from build123d import *

# Parameters (mm, degrees)
F0_R     = 12.7
F1_DEPTH = 12.7
F2_R     = 3.2385
F3_DEPTH = 12.7
F4_R     = 1.905
F5_DEPTH = 12.7


with BuildPart() as f1:
    # F0 (on Front) → F1 (new body)
    with BuildSketch(Plane.XZ):
        Circle(F0_R)
    extrude(amount=F1_DEPTH)

    # F2 (on face) → F3 (cut)
    with BuildSketch(Plane.XZ.offset(12.7)):
        Circle(F2_R)
    extrude(amount=-F3_DEPTH, mode=Mode.SUBTRACT)

    # F4 (on face) → F5 (join)
    with BuildSketch(Plane.XZ.offset(12.7)):
        with Locations((-8.480146, 3.001869)):
            Circle(F4_R)
        with Locations((-5.475456, -7.13747)):
            Circle(F4_R)
        with Locations((5.096128, -7.413068)):
            Circle(F4_R)
        with Locations((8.625037, 2.555942)):
            Circle(F4_R)
        with Locations((0.234438, 8.992727)):
            Circle(F4_R)
    extrude(amount=F5_DEPTH)


solid = f1.part
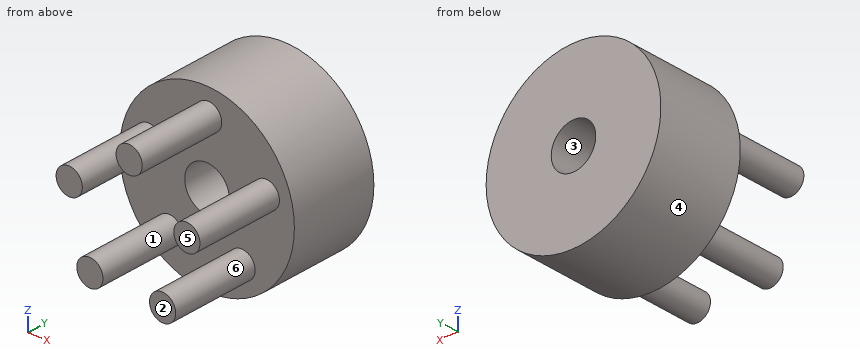
Model file for the job. Use its own axes, mm. Face numbers are marked on the shaded views. A direction names the side the tool comes from. Give positions to 0.01 mm unless a question says otherwise; leave off trailing zeros. Order: outer loops, then holes, each group sorted by start corner. A loop starts at its lowest first (then second) coordinate and runs counter-clockwise, first axis right, second up. Notation, with made-up numbers: M 57,27 L 65,27 A7 ccw 65,40 Z; hole C -31,47.5 d9. An arc over 180 degrees is marked long. Write item = value, one per line.
Q1. Cut at D-D, the plane y = -16.25. List the corners of the cut face in (x, z) (3 decimals).
Derived:
outline = C -8.48,3.002 d3.81; C -5.475,-7.137 d3.81; C 0.234,8.993 d3.81; C 5.096,-7.413 d3.81; C 8.625,2.556 d3.81
Q2. Cut at B-B, the plane x = 0. List the corners of the cut face in (y, z), then the cut area to 3 significant figures.
Derived:
outline = M -25.4,7.1 L -12.7,7.1 L -12.7,3.24 L 0,3.24 L 0,12.7 L -12.7,12.7 L -12.7,10.88 L -25.4,10.88 Z; M -12.7,-12.7 L 0,-12.7 L 0,-3.24 L -12.7,-3.24 Z
area = 288 mm2
Q3. Cut at A-A, the plane z = 0. List the corners of the cut face in (x, y), then the cut area to 3 significant figures.
Derived:
outline = M -12.7,-12.7 L -3.24,-12.7 L -3.24,0 L -12.7,0 Z; M 3.24,-12.7 L 12.7,-12.7 L 12.7,0 L 3.24,0 Z
area = 240 mm2
Q4. Two-plate mould, pull along Z, no slides. Class the marked faces 1, 2, 3 and 4: pulls with the +Z half, pulls with the -Z half, needs draft (parallel to the pull), parting line crosses it, or undercut.
Derived:
face_1 = undercut
face_2 = needs draft
face_3 = undercut
face_4 = parting line crosses it
Q5. Flat gauge pins, fed straight in: pin 1 (5 mm diameter, centred on x = 5.5, y = -15.5, fed in from -Z); pin 2 (3 mm diameter, centred on y = -12.5, z = -6.5, fed in from -X); pin 3 (6 mm diameter, centred on x = 8, y = -12.5, fed in from -Z). Where does each tip first touch, or does it go through?
Derived:
pin_1 = -9.32
pin_2 = -11.67
pin_3 = -11.67
Q6. Drill centre lines: line 1 (X direction, y = -19, z = -7.25); line 2 (Z direction, x = 0, y = -6); line 3 (X direction, y = -21, z = -8.25). Where is each one in solid material? Low to high. Write a range as [from, to].
Derived:
line_1 = [-7.38, -3.57], [3.2, 6.99]
line_2 = [-12.7, -3.24], [3.24, 12.7]
line_3 = [-7.02, -3.93], [3.38, 6.81]
Q7. Cut at C-C, the plane y = -9.75. List the corners of the cut face in (x, z), then the cut area to 3 significant figures.
Derived:
outline = C 0,0 d25.4; hole C 0,0 d6.48
area = 474 mm2
Q8. Tool access for the marked faces 5 and 6: list every direction of +Z, -Z, +X, -X, +Y, -Y with a clear straight run to the whole face (end or side of a thin tool).
Derived:
face_5 = +Z, -Z, +X, -X, -Y
face_6 = -Y
